Here's how the part is built. I have some questions about the finished solid (model axes, mm). A direction names the side the tool comes from. Give positions to 0.01 mm unless a question says otherwise; leave off trailing zeros. Loops run counter-clockwise (first coordinate to the right, second up) from the corner with the lowest first, then second, coordinate; pieces in that order, holes last.
Q1. If we section it at B-B (z = 0): Please give me the cut outline in (x, y) (3 decimals).
Q2. For faces 5 (the face through (38.1, 2, 0)), 6 (the face through (-27, 3.175, 0)), 7 (the face through (6.35, 35, 0)), which set-ups out of +Z, -Z, +X, -X, +Y, -Y let a thin tool reach every point of the face, with its end or its side?
Q3. We'd pull the mould along X, two halves only. Please class faces 1 (the face through (29.406, 1.252, -0.738)), 2 (the face through (-6.35, 35, 0)), 3 (the face through (0.32, 23.52, -0.38)), 4 (the face through (28, 3.175, 0)): +X half, -X half, draft (parallel to the pull), parting line (faces both ways), or undercut.
Q4. I need wall thicknesses on line 1 (Y direction, x = 0, z = 1) (3 decimals); line 2 (Z direction, x = 31.75, y = 1.6); line 3 (X direction, y = 19, z = 2.75). Which ranges of each line are inside material? Lowest first, please.
Q5. Will these pins go through, and if not, where does the flat tip stop? P1, Ø5, axis at y = 18.5, z = 0, coming from the -X side; P2, Ø2.5, axis at y = 37.5, z = -1.5, coming from the +X side; P3, Ø4, axis at y = 26.5, z = 3, coming from the +X side.
Q6. If we section it at A-A (x = 0): Please give me the cut outline in (y, z) (3 decimals).
Q7. If we section it at C-C (y = 35): Please give me the cut outline in (x, z), plus the area to 3 significant figures.
Q8. If we section it at D-D (x = -31.75): Please give me the cut outline in (y, z) (3 decimals), plus the area to 3 significant figures.
from build123d import *

# Parameters (mm, degrees)
SKETCH1_W                       = 76.2
SKETCH1_H                       = 9.144
BOSS_EXTRUDE1_DEPTH             = 3.175
F_8_CLEARANCE_HOLE1_D           = 4.9149
F_8_CLEARANCE_HOLE1_CSINK_D     = 6.1849
F_8_CLEARANCE_HOLE1_CSINK_ANGLE = 90
BOSS_EXTRUDE2_DEPTH             = 9.144
F_8_CLEARANCE_HOLE2_D           = 4.9149
F_8_CLEARANCE_HOLE2_CSINK_D     = 6.1849
F_8_CLEARANCE_HOLE2_CSINK_ANGLE = 90


with BuildPart() as part:
    # Sketch1 → Boss-Extrude1 (new body)
    with BuildSketch(Plane(origin=(0, 0, 0), x_dir=(1, 0, 0), z_dir=(0, 1, 0))):
        Rectangle(SKETCH1_W, SKETCH1_H)
    extrude(amount=BOSS_EXTRUDE1_DEPTH)

    # #8 Clearance Hole1 (through all)
    with Locations(Plane(origin=(0, 3.175, 0), x_dir=(1, 0, 0), z_dir=(0, 1, 0))):
        with Locations((-31.75, 0), (31.75, 0)):
            CounterSinkHole(F_8_CLEARANCE_HOLE1_D / 2, F_8_CLEARANCE_HOLE1_CSINK_D / 2, counter_sink_angle=F_8_CLEARANCE_HOLE1_CSINK_ANGLE)

    # Sketch4 → Boss-Extrude2 (add)
    with BuildSketch(Plane.XY.offset(4.572)):
        Polygon((-6.35, 28.575), (-19.05, 3.175), (0, 3.175), (0, 41.275), (-6.35, 41.275), align=None)
        Polygon((0, 41.275), (0, 3.175), (19.05, 3.175), (6.35, 28.575), (6.35, 41.275), align=None)
    extrude(amount=-BOSS_EXTRUDE2_DEPTH)

    # #8 Clearance Hole2 (through all)
    with Locations(Plane.XY.offset(4.572)):
        with Locations((0, 21.082)):
            CounterSinkHole(F_8_CLEARANCE_HOLE2_D / 2, F_8_CLEARANCE_HOLE2_CSINK_D / 2, counter_sink_angle=F_8_CLEARANCE_HOLE2_CSINK_ANGLE)


solid = part.part
Check sheet entries:
1. outline: (-38.1, 0) - (-34.207, 0) - (-34.207, 2.54) - (-34.842, 3.175) - (-38.1, 3.175) - close; (-29.293, 0) - (29.293, 0) - (29.293, 2.54) - (28.658, 3.175) - (19.05, 3.175) - (6.35, 28.575) - (6.35, 41.275) - (-6.35, 41.275) - (-6.35, 28.575) - (-19.05, 3.175) - (-28.658, 3.175) - (-29.293, 2.54) - close; (34.207, 0) - (38.1, 0) - (38.1, 3.175) - (34.842, 3.175) - (34.207, 2.54) - close; hole circle Ø4.915 at (0, 21.082)
2. face 5: +Z, -Z, +X, +Y, -Y
2. face 6: +Z, -Z, -X, +Y
2. face 7: +Z, -Z, +X, +Y
3. face 1: undercut
3. face 2: -X half
3. face 3: undercut
3. face 4: draft
4. line 1: y = 0 to 18.625, 23.539 to 41.275
4. line 2: z = -4.57 to -2.46, 2.46 to 4.57
4. line 3: x = -11.14 to -1.31, 1.31 to 11.14
5. P1: stops at x = -12.64
5. P2: stops at x = 6.35
5. P3: stops at x = 8.39
6. outline: (0, -4.572) - (18.625, -4.572) - (18.625, 3.937) - (17.99, 4.572) - (0, 4.572) - close; (23.539, -4.572) - (41.275, -4.572) - (41.275, 4.572) - (24.174, 4.572) - (23.539, 3.937) - close
7. outline: (-6.35, -4.57) - (6.35, -4.57) - (6.35, 4.57) - (-6.35, 4.57) - close
7. area: 116 mm2
8. outline: (0, -4.572) - (3.175, -4.572) - (3.175, -3.092) - (2.54, -2.457) - (0, -2.457) - close; (0, 2.457) - (2.54, 2.457) - (3.175, 3.092) - (3.175, 4.572) - (0, 4.572) - close
8. area: 13.0 mm2
